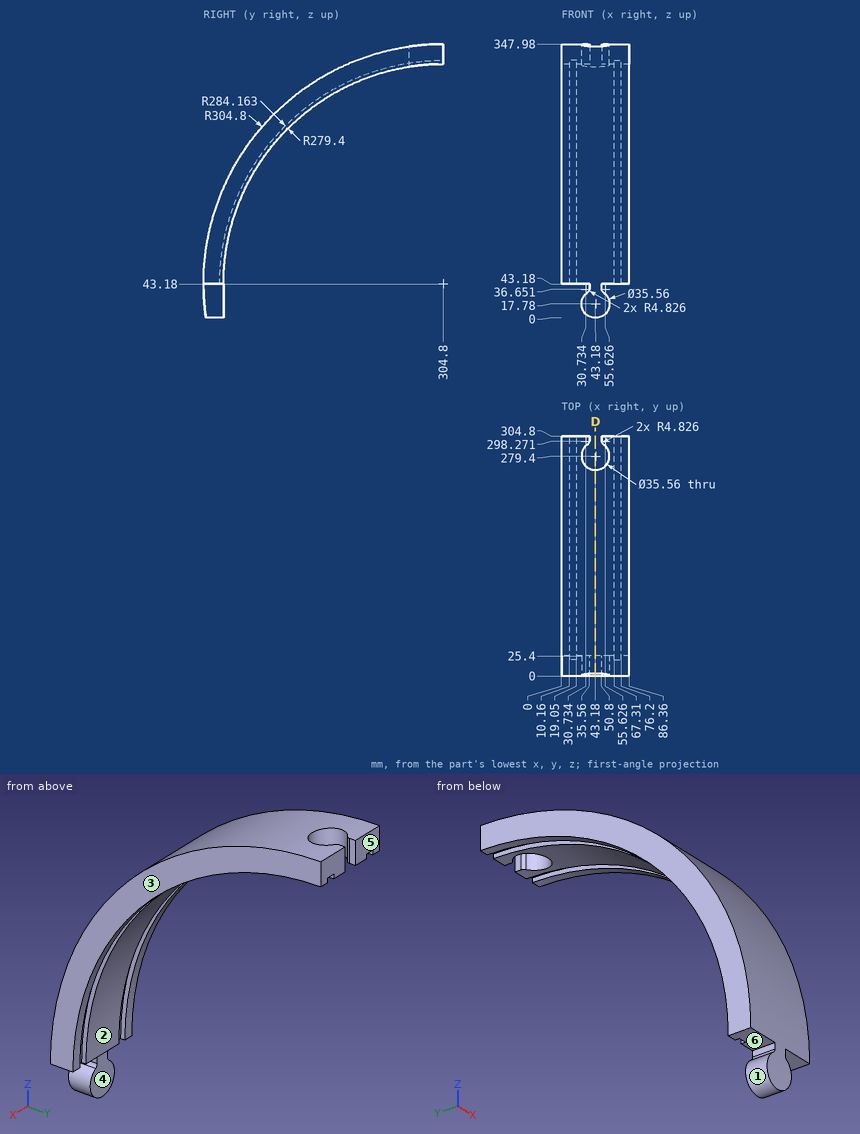
Design review of the part shown in the three views and the two pictorial views. Dimensions are in mm from the part's minimum x, y and z. A direction names the side the tool comes from. Give positions to 0.01 mm unless a question says otherwise; leave off trailing zeros. Loops run counter-clockwise (first coordinate to the right, second up) from the corner with the lowest first, then second, coordinate; pieces in that order, holes last. Notation, with made-up numbers: (-31, -11) -> (-26, -11) arc R7 cw to (-26, -7) -> close; hole circle Ø2 at (-4, 4). An arc over 180 degrees is marked (long way). Put each result on its own line as item: value. Start each with the question number.
1. Wall thickness on probe 1 along X at (y, z) = (279.4, 326); probe 2 along X at (y, z) = (279, 337) (1 decimal); probe 3 along Z at (x, y) = (44.5, 235): over which ranges is each line inside the solid? List them lowest first.
2. Clearance check with flat-ended pins moving along their axes: P1, Ø18, axis at x = 46.5, z = 30.5, coming from the +Y side; P2, Ø10, axis at x = 10.5, y = 261.5, coming from the +Z side; P3, Ø2, axis at y = 16.5, z = 40, coming from the +X side. State where each tip first meets the part, or that it passes through.
3. We need section D-D on x = 43.18. State the section outline as (y, z) points (1 decimal), then the cut area to 3 significant figures.
4. Mouldability with a two-part tool opening along Z and no side actions: class the marked faces 1, 2 and 3 as released by +Z, released by -Z, zero draft, split by the parting line, or undercut.
5. For the marked faces 4, 5 and 6, list the 3-axis set-ups (+Z, -Z, +X, -X, +Y, -Y) from which the entire face can be reached by the end or side of a thin tool; tool diameter is ignored.
Determined:
1. probe 1: 0 to 10.16, 19.05 to 25.4, 60.96 to 67.31, 76.2 to 86.36
1. probe 2: 0 to 25.4, 61 to 86.4
1. probe 3: 313.72 to 339.88
2. P1: y = 25.4
2. P2: z = 345.56
2. P3: x = 50.8
3. outline: (3.1, 0) -> (25.4, 0) -> (25.4, 43.2) arc R279.4 cw to (261.6, 319.2) -> (261.6, 344.9) arc R304.8 ccw to start
3. area: 11,600 mm^2
4. face 1: undercut
4. face 2: released by -Z
4. face 3: zero draft
5. face 4: -Z, +X, -X, +Y
5. face 5: +Z, -Z, +X, -X, +Y
5. face 6: -X, +Y, -Y
